Build history of the part. All positions in model axes, mm. A direction names the side the tool comes from. Give positions to 0.01 mm unless a question says otherwise; leave off trailing zeros. Write each loop counter-clockwise with the first axis right and the second up, starting at its lowest first coordinate (ties: lowest second). Pieces come first, ordered by that corner, then holes. Notation, with made-up numbers: (-28.5, -16.75) -> (-23.5, -16.75) arc R17 ccw to (-23.5, 0.25) -> close; hole circle Ø5 at (74.25, -2.75). An arc over 180 degrees is marked (long way). Put each result on its own line as item: value.
from build123d import *

# Parameters (mm, degrees)
SKETCH1_R                       = 25.4
SKETCH1_R_2                     = 13.49375
BOSS_EXTRUDE1_DEPTH             = 19.05
F_8_0_199_DIAMETER_HOLE1_REACH  = 61.906
F_8_0_199_DIAMETER_HOLE1_BORE_R = 2.5273
BULKHEAD_THROUGH_REACH          = 66.212
BULKHEAD_THROUGH_END_RADIUS     = 13.49375
SKETCH6_R                       = 2.667
SKETCH6_4_R                     = 5.207
ACCESS_HOLE_DEPTH               = 6.35
CIRPATTERN1_COUNT               = 4


with BuildPart() as part:
    # Sketch1 → Boss-Extrude1 (new body)
    with BuildSketch(Plane(origin=(0, 0, 0), x_dir=(1, 0, 0), z_dir=(0, 1, 0))):
        with Locations(Location((0, 0, 0), (0, 0, 90))):
            Circle(SKETCH1_R)
        with Locations(Location((0, 0, 0), (0, 0, 90))):
            Circle(SKETCH1_R_2, mode=Mode.SUBTRACT)
    extrude(amount=BOSS_EXTRUDE1_DEPTH)

    # #8 (0.199) Diameter Hole1 bore → #8 (0.199) Diameter Hole1 (cut, up to next)
    with BuildSketch(Plane(origin=(25.4, 0, 0), x_dir=(0, 0, -1), z_dir=(1, 0, 0)), mode=Mode.PRIVATE) as f_8_0_199_diameter_hole1_sk1:
        with Locations((0, 9.525)):
            Circle(F_8_0_199_DIAMETER_HOLE1_BORE_R)
    f_8_0_199_diameter_hole1_tool1 = extrude(f_8_0_199_diameter_hole1_sk1.sketch, amount=-F_8_0_199_DIAMETER_HOLE1_REACH, mode=Mode.PRIVATE) & part.part
    f_8_0_199_diameter_hole1 = f_8_0_199_diameter_hole1_tool1.solids().sort_by_distance((25.4, 9.525, 0))[0]
    add(f_8_0_199_diameter_hole1, mode=Mode.SUBTRACT)

    # bulkhead_through: up to this cylinder (the profile starts outside it)
    bulkhead_through_end = Plane(origin=(0, 9.525, 0), z_dir=(0, -1, 0)) * Cylinder(BULKHEAD_THROUGH_END_RADIUS, 160.4115, mode=Mode.PRIVATE)
    # Sketch6 → bulkhead_through (cut, up to the surface)
    with BuildSketch(Plane(origin=(17.960512242, 0, 17.960512242), x_dir=(0.7071067811865487, 0, -0.7071067811865465), z_dir=(0.7071067811865465, 0, 0.7071067811865487)), mode=Mode.PRIVATE) as bulkhead_through_sk1:
        with Locations((0, 9.525)):
            Circle(SKETCH6_R)
    bulkhead_through_tool1 = extrude(bulkhead_through_sk1.sketch, amount=-BULKHEAD_THROUGH_REACH, mode=Mode.PRIVATE) - bulkhead_through_end
    bulkhead_through = bulkhead_through_tool1.solids().sort_by_distance((17.960512, 9.525, 17.960512))[0]
    add(bulkhead_through, mode=Mode.SUBTRACT)

    # Sketch6<4> → access_hole (cut)
    with BuildSketch(Plane(origin=(17.960512242, 0, 17.960512242), x_dir=(0.7071067811865487, 0, -0.7071067811865465), z_dir=(0.7071067811865465, 0, 0.7071067811865487))):
        with Locations((0, 9.525)):
            Circle(SKETCH6_4_R)
    access_hole = extrude(amount=-ACCESS_HOLE_DEPTH, mode=Mode.SUBTRACT)

    # CirPattern1: #8 (0.199) Diameter Hole1, bulkhead_through, access_hole ×4 about axis
    cirpattern1_axis = Axis((0, 0, 0), (0, 1, 0))
    add([f_8_0_199_diameter_hole1.rotate(cirpattern1_axis, i * 360 / CIRPATTERN1_COUNT) for i in range(1, CIRPATTERN1_COUNT)], mode=Mode.SUBTRACT)
    add([bulkhead_through.rotate(cirpattern1_axis, i * 360 / CIRPATTERN1_COUNT) for i in range(1, CIRPATTERN1_COUNT)], mode=Mode.SUBTRACT)
    add([access_hole.rotate(cirpattern1_axis, i * 360 / CIRPATTERN1_COUNT) for i in range(1, CIRPATTERN1_COUNT)], mode=Mode.SUBTRACT)


solid = part.part
1) Slice it at A-A (z = 0). Write the cut outline in (x, y).
Filled sheet:
outline: (-25.4, 0) -> (-13.49, 0) -> (-13.49, 7) -> (-25.4, 7) -> close; (-25.4, 12.05) -> (-13.49, 12.05) -> (-13.49, 19.05) -> (-25.4, 19.05) -> close; (13.49, 0) -> (25.4, 0) -> (25.4, 7) -> (13.49, 7) -> close; (13.49, 12.05) -> (25.4, 12.05) -> (25.4, 19.05) -> (13.49, 19.05) -> close
2) Pull direction Z, two halves, no side cores. Call faces 1 (the cylindrical face through (9.728, 9.392, -23.463)), 2 (the cylindrical face through (10.427, 11.774, -12.454)), 3 (the flat face through (11, 0, -11)): released by +Z, released by -Z, zero draft, split by the parting line, or undercut.
Filled sheet:
face 1: split by the parting line
face 2: undercut
face 3: zero draft
3) Slice it at B-B (x = 0). Write the cut outline in (y, z).
Filled sheet:
outline: (0, -25.4) -> (7, -25.4) -> (7, -13.49) -> (0, -13.49) -> close; (0, 13.49) -> (7, 13.49) -> (7, 25.4) -> (0, 25.4) -> close; (12.05, -25.4) -> (19.05, -25.4) -> (19.05, -13.49) -> (12.05, -13.49) -> close; (12.05, 13.49) -> (19.05, 13.49) -> (19.05, 25.4) -> (12.05, 25.4) -> close
4) Wall check: L1, parallel to Z at x = -10.5, y = 8.5; L2, parallel to Z at x = 11, y = 13.25; L3, parallel to Z at x = 0, y = 15.75. Give the ranges that are in metal, low to high.
Filled sheet:
L1: -23.13 to -17.72, -16.44 to -13.98, 13.98 to 16.44, 17.72 to 23.13
L2: -22.89 to -16.15, -15.94 to -7.82, 7.82 to 15.94, 16.15 to 22.89
L3: -25.4 to -13.49, 13.49 to 25.4
5) Slice it at C-C (y = 6). Write the cut outline in (x, z).
Filled sheet:
outline: (-20.46, -15.04) -> (-16.18, -10.76) -> (-10.76, -16.18) -> (-15.04, -20.46) arc R25.4 ccw to (15.04, -20.46) -> (10.76, -16.18) -> (16.18, -10.76) -> (20.46, -15.04) arc R25.4 ccw to (20.46, 15.04) -> (16.18, 10.76) -> (10.76, 16.18) -> (15.04, 20.46) arc R25.4 ccw to (-15.04, 20.46) -> (-10.76, 16.18) -> (-16.18, 10.76) -> (-20.46, 15.04) arc R25.4 ccw to start; hole circle Ø26.99 at (0, 0)
6) Slice it at D-D (y = 2.25). Write the cut outline in (x, z), plus the area to 3 significant figures.
Filled sheet:
outline: circle Ø50.8 at (0, 0); hole circle Ø26.99 at (0, 0)
area: 1,450 mm2
7) Pin check, flat tips, straight feed: pin 1 (3 mm diameter, centred on x = 9, y = 8, fed in from +Z); pin 2 (8 mm diameter, centred on x = -17.5, y = 11, fed in from +Z); pin 3 (2 mm diameter, centred on y = 2, z = 3.5, fed in from +X). Stop position of each tip, or through.
Filled sheet:
pin 1: z = 24.27
pin 2: z = 21.52
pin 3: x = 25.28
8) Tool access for faces 4 (the flat face through (15.055, 7.284, 11.886)), 5 (the cylindrical face through (5.168, 9.392, -12.465)): list every direction of +Z, -Z, +X, -X, +Y, -Y with a clear straight run to the whole face (end or side of a thin tool).
Filled sheet:
face 4: none
face 5: +Y, -Y
